Autodesk Inventor part; units mm, degrees
ref_plane "YZ Plane" through (0, 0, 0) normal (1, 0, 0) x (0, 1, 0)
ref_plane "XZ Plane" through (0, 0, 0) normal (0, 1, 0) x (-1, 0, 0)
ref_plane "XY Plane" through (0, 0, 0) normal (0, 0, 1) x (1, 0, 0)
sketch "Sketch1" plane through (0, 0, 0) normal (0, 1, 0) x (-1, 0, 0)
  line L0 (2.1273, 2.1273) -> (-2.1273, 2.1273)
  line L1 (-2.1273, 2.1273) -> (-2.1273, -2.1273)
  line L2 (-2.1273, -2.1273) -> (2.1273, -2.1273)
  line L3 (2.1273, -2.1273) -> (2.1273, 2.1273)
  circle A0 centre (0, 0) radius 9.525
  point P0 (2.1273, 0)
  point P1 (0, -2.1272)
  dimension "d0" = 4.2545
  dimension "d1" = 19.05
extrude "Extrusion1" add sketch "Sketch1" along normal blind 9.525
sketch "Sketch2" plane through (0, 0, 0) normal (0, -1, 0) x (1, 0, 0)
  line L0 (-4.7625, 2.7496) -> (0, 5.4993)
  line L1 (0, 5.4993) -> (4.7625, 2.7496)
  line L2 (4.7625, 2.7496) -> (4.7625, -2.7496)
  line L3 (4.7625, -2.7496) -> (0, -5.4993)
  line L4 (0, -5.4993) -> (-4.7625, -2.7496)
  line L5 (-4.7625, -2.7496) -> (-4.7625, 2.7496)
  circle A0 centre (0, 0) radius 9.525
  dimension "d4" = 9.525
extrude "Extrusion2" add sketch "Sketch2" along normal blind 9.525
sketch "Sketch3" plane through (0, 0, 0) normal (1, 0, 0) x (0, 1, 0)
  circle A0 centre (-4.7625, 0) radius 2.4447
  circle A1 centre (4.7625, -0.254) radius 2.4447
  line L0 (0, 2.1273) -> (9.525, 2.1273)
  line L1 (0, 2.7496) -> (-9.525, 2.7496)
  point P0 (0, 0)
  point P1 (-4.7625, 2.7496)
  point P2 (4.7625, 2.1273)
  dimension "d7" = 4.8895
  dimension "d8" = 4.8895
extrude "Extrusion3" cut sketch "Sketch3" along normal mid plane 19.05
Verification items for the finished model (mm, model axes). A direction names the side the tool comes from. Give positions to 0.01 mm unless a question says otherwise; leave off trailing zeros. Write each loop counter-clockwise with the first axis right and the second up, starting at its lowest first coordinate (ties: lowest second). Pieces come first, ordered by that corner, then holes. Notation, with made-up numbers: M 24.25,68 L 78.25,68 A11 ccw 78.25,78 Z; hole C 35,-30.5 d4. An arc over 180 degrees is marked long. Put each result on its own line as item: value. Start each with the question number.
1. Section check B-B (x = 1.5). Record the cut outline in (y, z) (1 decimal).
2. Draft check along Y on faces 4 (the face through (4.762, -3.6, 2.5)), 5 (the face through (-2.3, -9.525, 4.4)), 6 (the face through (-7.11, -2.43, 0.73)). Enter one of: +Y half, -Y half, draft (parallel to the pull), parting line (faces both ways), or undercut.
3. Scan lines: line 1 along Y through (x, z) = (6.1, 0) (3 decimals); line 2 along Y through (x, z) = (-5.5, -2) (3 decimals); line 3 along Z through (x, y) = (8.25, -0.5). Record each from-to range of solid material in increasing order. Write a range as [from, to].
4. Set-up check for faces 1 (the face through (0.1, 9.525, 2.3)), 2 (the face through (0, 2, 2.127)), 3 (the face through (-2.348, -4.696, -4.144)): record each of +Z, -Z, +X, -X, +Y, -Y from which the full face is reachable in a straight line by a thin tool's end or side.
5. Section check C-C (z = -1.75). Record the cut outline in (x, y) (1 decimal), and give its area (3 significant figures).
6. Go/stop test with flat-tipped pins: pin 1 Ø1.5 at (x, y) = (6.5, -3) entering from -Z; pin 2 Ø7.5 at (x, z) = (-0.5, 0.5) entering from -Y; pin 3 Ø6 at (y, z) = (0.5, 5.5) entering from +X; pin 4 Ø3 at (y, z) = (-4.76, 0) entering from -X. Record where each tip stops, or that it passes through.
7. Section check D-D (x = 7.75). Record the cut outline in (y, z) (1 decimal).
Answer list:
1. outline: M -9.5,-9.4 L 9.5,-9.4 L 9.5,-2.1 L 6.3,-2.1 A2.4 cw 3.2,-2.1 L 0,-2.1 L 0,-4.6 L -9.5,-4.6 Z; M -9.5,4.6 L 0,4.6 L 0,2.1 L 4.2,2.1 A2.4 cw 5.3,2.1 L 9.5,2.1 L 9.5,9.4 L -9.5,9.4 Z
2. face 4: draft
2. face 5: -Y half
2. face 6: undercut
3. line 1: [-9.525, -7.207], [-2.318, 2.331], [7.194, 9.525]
3. line 2: [-9.525, -6.168], [-3.357, 3.051], [6.474, 9.525]
3. line 3: [-4.76, 4.76]
4. face 1: +Z, -Z, +X, -X, +Y
4. face 2: +Y, -Y
4. face 3: -Y
5. outline: M -9.4,-9.5 L -4.8,-9.5 L -4.8,-6.5 L -9.4,-6.5 Z; M -9.4,-3.1 L -4.8,-3.1 L -4.8,0 L -2.1,0 L -2.1,2.8 L -9.4,2.8 Z; M -9.4,6.7 L -2.1,6.7 L -2.1,9.5 L -9.4,9.5 Z; M 2.1,0 L 4.8,0 L 4.8,-3.1 L 9.4,-3.1 L 9.4,2.8 L 2.1,2.8 Z; M 2.1,6.7 L 9.4,6.7 L 9.4,9.5 L 2.1,9.5 Z; M 4.8,-9.5 L 9.4,-9.5 L 9.4,-6.5 L 4.8,-6.5 Z
5. area: 138 mm2
6. pin 1: z = -7.59
6. pin 2: y = 0
6. pin 3: x = 9.19
6. pin 4: through
7. outline: M -9.5,-5.5 L 9.5,-5.5 L 9.5,5.5 L -9.5,5.5 Z; hole C -4.8,0 d4.9; hole C 4.8,-0.3 d4.9
